Can you work these out from the model? Positions are in its coordinate system, mm. Coordinates: 2 decimals unless noted, no trailing zeros. Loops run counter-clockwise (first coordinate to the right, second up) from the corner with the lowest first, then second, coordinate; pieces in that order, holes last.
```python
from build123d import *

# Parameters (mm, degrees)
SKETCH_1_W          = 10
SKETCH_1_H          = 16
SKETCH_1_R          = 1.5
EXTRUDE_1_DEPTH     = 10
CUT_EXTRUDE_1_DEPTH = 10
SKETCH_3_R          = 3
CUT_EXTRUDE_2_DEPTH = 22.65119524


with BuildPart() as part:
    # 草图1 → 凸台-拉伸1 (new body)
    with BuildSketch(Plane(origin=(0, 0, 0), x_dir=(1, 0, 0), z_dir=(0, 1, 0))):
        with Locations((5, 8)):
            Rectangle(SKETCH_1_W, SKETCH_1_H)
        with Locations(Location((5, 10, 0), (0, 0, 270))):
            Circle(SKETCH_1_R, mode=Mode.SUBTRACT)
    extrude(amount=EXTRUDE_1_DEPTH)

    # 草图2 → 切除-拉伸1 (cut)
    with BuildSketch(Plane(origin=(10, 0, 0), x_dir=(0, 0, -1), z_dir=(1, 0, 0))):
        Polygon((0, 1.43111196), (6, 10), (0, 10), align=None)
    extrude(amount=-CUT_EXTRUDE_1_DEPTH, mode=Mode.SUBTRACT)

    # 草图3 → 切除-拉伸2 (cut, through all)
    with BuildSketch(Plane(origin=(0, 0.470821421, 0.672402674), x_dir=(1, 0, 0), z_dir=(0, 0.5735764363510438, 0.8191520442889935))):
        with Locations(Location((5, 6.402638674, 0), (0, 0, 270))):
            Circle(SKETCH_3_R)
    extrude(amount=-CUT_EXTRUDE_2_DEPTH, mode=Mode.SUBTRACT)


solid = part.part
```
Item 1: Suppose I cut it at C-C, the plane x = 5. Please give me the cut outline in (y, z), plus the area to 3 significant figures.
Results are:
outline: (0, -5.93) - (3.26, -1.28) - (1.43, 0) - (0, 0) - close; (0.28, -16) - (10, -16) - (10, -11.5) - (3.43, -11.5) - close; (5.53, -8.5) - (10, -8.5) - (10, -6) - (8.17, -4.72) - close
area: 58.0 mm2
Item 2: Suppose I cut it at B-B, the plane x = 7.25. Please give me the cut outline in (y, z).
Results are:
outline: (0, -16) - (10, -16) - (10, -6) - (7.34, -4.14) - (0, -14.62) - close; (0, -7.7) - (4.09, -1.86) - (1.43, 0) - (0, 0) - close
Item 3: Suppose I cut it at A-A, the plane x = 1. Please give me the cut outline in (y, z).
Results are:
outline: (0, -16) - (10, -16) - (10, -6) - (1.43, 0) - (0, 0) - close
Item 4: We'd pull the mould along Z, two halves only. Please class faces 1 (the face through (5, 1, 0)), 2 (the face through (7.028, 4.476, -8.625)), 3 (the face through (0, 5, -10)): +Z half, -Z half, draft (parallel to the pull), parting line (faces both ways), or undercut.
Results are:
face 1: +Z half
face 2: undercut
face 3: draft
Item 5: I'm going to push flat-ended pins straight in: P1, Ø1.8, axis at x = 5, z = -10, coming from the -Y side; P2, Ø6, axis at x = 8, y = 4.5, coming from the +Z side. Where does each tip first touch, or does it pass through?
Results are:
P1: passes through
P2: stops at z = -0.05
Item 6: I need wall thicknesses on line 1 along X through (y, z) = (8.75, -10); line 2 along Z through (x, y) = (5, 8); line 3 along Z through (x, y) = (5, 6). Which ranges of each line are inside material? Lowest first, please.
Results are:
line 1: x = 0 to 3.5, 6.5 to 10
line 2: z = -16 to -11.5, -8.5 to -4.97
line 3: z = -16 to -11.5, -8.5 to -7.82
Item 7: Suppose I cut it at D-D, the plane y = 8.75. Please give me the cut outline in (x, z).
Results are:
outline: (0, -16) - (10, -16) - (10, -5.12) - (0, -5.12) - close; hole circle Ø3 at (5, -10)
